Work out the finished part from the listing and answer in its coordinate system (mm). A direction names the side the tool comes from. Coordinates: 2 decimals unless noted, no trailing zeros. Write each loop counter-clockwise with the first axis right and the second up, starting at its lowest first coordinate (ties: lowest second). Pieces come first, ordered by that corner, then holes. Notation, with made-up numbers: (31, 35) - (72, 35) arc R11 ccw to (72, 48) - close; hole circle Ø3 at (58.5, 81). An arc over 180 degrees is marked (long way). One line per item, written item: value.
```python
from build123d import *

# Parameters (mm, degrees)
SKETCH2_W           = 40.6
SKETCH2_H           = 36.6
SKETCH2_W_2         = 6.4
SKETCH2_H_2         = 2.4
SKETCH2_W_3         = 5.8
SKETCH2_H_3         = 5.3
BOSS_EXTRUDE1_DEPTH = 19.8
CUT_EXTRUDE1_DEPTH  = 5.3
CUT_EXTRUDE2_DEPTH  = 30.3


with BuildPart() as part:
    # Sketch2 → Boss-Extrude1 (new body)
    with BuildSketch(Plane(origin=(0, 0, 0), x_dir=(0, 0, -1), z_dir=(1, 0, 0))):
        Rectangle(SKETCH2_W, SKETCH2_H)
        with Locations((-23.5, 9.8)):
            Rectangle(SKETCH2_W_2, SKETCH2_H_2)
        with Locations((9.9, 20.95)):
            Rectangle(SKETCH2_W_3, SKETCH2_H_3)
        with Locations((23.5, 9.8)):
            Rectangle(SKETCH2_W_2, SKETCH2_H_2)
    extrude(amount=BOSS_EXTRUDE1_DEPTH)

    # Sketch3 → Cut-Extrude1 (cut)
    with BuildSketch(Plane(origin=(0, 18.3, 0), x_dir=(1, 0, 0), z_dir=(0, 1, 0))):
        with BuildLine():
            Line((9.9, 7), (12.8, 7))
            Line((12.8, 7), (12.8, 9.9))
            ThreePointArc((12.8, 9.9), (11.950609665, 7.849390335), (9.9, 7))
        make_face()
        with BuildLine():
            ThreePointArc((9.9, 12.8), (11.950609665, 11.950609665), (12.8, 9.9))
            Line((12.8, 9.9), (12.8, 12.8))
            Line((12.8, 12.8), (9.9, 12.8))
        make_face()
        with BuildLine():
            ThreePointArc((7, 9.9), (7.849390335, 11.950609665), (9.9, 12.8))
            Line((9.9, 12.8), (7, 12.8))
            Line((7, 12.8), (7, 9.9))
        make_face()
        with BuildLine():
            Line((7, 7), (9.9, 7))
            ThreePointArc((9.9, 7), (7.849390335, 7.849390335), (7, 9.9))
            Line((7, 9.9), (7, 7))
        make_face()
        Polygon((0, 7), (7, 7), (7, 9.9), (7, 12.8), (0, 12.8), align=None)
        Polygon((12.8, 7), (19.8, 7), (19.8, 12.8), (12.8, 12.8), (12.8, 9.9), align=None)
    extrude(amount=CUT_EXTRUDE1_DEPTH, mode=Mode.SUBTRACT)

    # Sketch4 → Cut-Extrude2 (cut, through all)
    with BuildSketch(Plane(origin=(0, 11, 0), x_dir=(1, 0, 0), z_dir=(0, 1, 0))):
        with BuildLine():
            ThreePointArc((16.4, 25.877050983), (14.9, 26.45), (13.4, 25.877050983))
            Line((13.4, 25.877050983), (16.4, 25.877050983))
        make_face()
        with BuildLine():
            Line((16.4, 25.877050983), (13.4, 25.877050983))
            ThreePointArc((13.4, 25.877050983), (13.981441346, 22.146040409), (17.15, 24.2))
            ThreePointArc((17.15, 24.2), (16.953959591, 25.118558654), (16.4, 25.877050983))
        make_face()
        with BuildLine():
            Line((16.4, 26.7), (13.4, 26.7))
            Line((13.4, 26.7), (13.4, 25.877050983))
            ThreePointArc((13.4, 25.877050983), (14.9, 26.45), (16.4, 25.877050983))
            Line((16.4, 25.877050983), (16.4, 26.7))
        make_face()
        with BuildLine():
            ThreePointArc((7.15, 24.2), (6.953959591, 25.118558654), (6.4, 25.877050983))
            Line((6.4, 25.877050983), (3.4, 25.877050983))
            ThreePointArc((3.4, 25.877050983), (3.981441346, 22.146040409), (7.15, 24.2))
        make_face()
        with BuildLine():
            Line((3.4, 25.877050983), (6.4, 25.877050983))
            ThreePointArc((6.4, 25.877050983), (4.9, 26.45), (3.4, 25.877050983))
        make_face()
        with BuildLine():
            Line((6.4, 25.877050983), (6.4, 26.7))
            Line((6.4, 26.7), (3.4, 26.7))
            Line((3.4, 26.7), (3.4, 25.877050983))
            ThreePointArc((3.4, 25.877050983), (4.9, 26.45), (6.4, 25.877050983))
        make_face()
        with BuildLine():
            ThreePointArc((13.4, -25.877050983), (14.9, -26.45), (16.4, -25.877050983))
            Line((16.4, -25.877050983), (13.4, -25.877050983))
        make_face()
        with BuildLine():
            Line((13.4, -25.877050983), (16.4, -25.877050983))
            ThreePointArc((16.4, -25.877050983), (16.953959591, -25.118558654), (17.15, -24.2))
            ThreePointArc((17.15, -24.2), (13.981441346, -22.146040409), (13.4, -25.877050983))
        make_face()
        with BuildLine():
            Line((13.4, -26.7), (16.4, -26.7))
            Line((16.4, -26.7), (16.4, -25.877050983))
            ThreePointArc((16.4, -25.877050983), (14.9, -26.45), (13.4, -25.877050983))
            Line((13.4, -25.877050983), (13.4, -26.7))
        make_face()
        with BuildLine():
            ThreePointArc((3.4, -25.877050983), (4.9, -26.45), (6.4, -25.877050983))
            Line((6.4, -25.877050983), (3.4, -25.877050983))
        make_face()
        with BuildLine():
            Line((3.4, -25.877050983), (6.4, -25.877050983))
            ThreePointArc((6.4, -25.877050983), (6.953959591, -25.118558654), (7.15, -24.2))
            ThreePointArc((7.15, -24.2), (3.981441346, -22.146040409), (3.4, -25.877050983))
        make_face()
        with BuildLine():
            Line((3.4, -26.7), (6.4, -26.7))
            Line((6.4, -26.7), (6.4, -25.877050983))
            ThreePointArc((6.4, -25.877050983), (4.9, -26.45), (3.4, -25.877050983))
            Line((3.4, -25.877050983), (3.4, -26.7))
        make_face()
    extrude(amount=-CUT_EXTRUDE2_DEPTH, mode=Mode.SUBTRACT)


solid = part.part
```
Item 1: Section A-A, the plane x = 1.5 is taken. Determine the outline of the cut face in (y, z).
Evaluation:
outline: (-18.3, -20.3) - (8.6, -20.3) - (8.6, -26.7) - (11, -26.7) - (11, -20.3) - (18.3, -20.3) - (18.3, 20.3) - (11, 20.3) - (11, 26.7) - (8.6, 26.7) - (8.6, 20.3) - (-18.3, 20.3) - close
Item 2: Section C-C, the plane z = 12 is taken. Determine the outline of the cut face in (x, y), then the cut area to 3 significant figures.
Evaluation:
outline: (0, -18.3) - (19.8, -18.3) - (19.8, 18.3) - (0, 18.3) - close
area: 725 mm2
Item 3: Given pin 1 (4 mm diameter, centred on x = 7.5, y = 17, fed in from -Z); pin 2 (1.9 mm diameter, centred on x = 13, z = -23, fed in from +Y); pin 3 (10 mm diameter, centred on x = 9, z = 9.5, fed in from +Y), each flat-ended and moving along its own axis, determine where each tip first touches the part or whether it passes through.
Evaluation:
pin 1: stops at z = -20.3
pin 2: stops at y = 11
pin 3: stops at y = 18.3
Item 4: Section B-B, the plane y = 21 is taken. Determine the outline of the cut face in (x, z), then the cut area to 3 significant figures.
Evaluation:
outline: circle Ø5.8 at (9.9, -9.9)
area: 26.4 mm2
Item 5: Section D-D, the plane x = 14.9 is taken. Determine the outline of the cut face in (y, z).
Evaluation:
outline: (-18.3, -20.3) - (8.6, -20.3) - (8.6, -21.95) - (11, -21.95) - (11, -20.3) - (18.3, -20.3) - (18.3, 20.3) - (11, 20.3) - (11, 21.95) - (8.6, 21.95) - (8.6, 20.3) - (-18.3, 20.3) - close
Item 6: Consider probe 1 along X at (y, z) = (9.7, 24.2); probe 2 along Z at (x, y) = (10.5, -2.5); probe 3 along Z at (x, y) = (4.9, 9.75). Determine where each line is inside the solid, lowest interval first.
Evaluation:
probe 1: x = 0 to 2.65, 7.15 to 12.65, 17.15 to 19.8
probe 2: z = -20.3 to 20.3
probe 3: z = -21.95 to 21.95
Item 7: Which of the six approach directions +Z, -Z, +X, -X, +Y, -Y give full straight-line access (tool end or side, diameter ignored) to faces 1 (the face through (10, 8.6, 24)), 2 (the face through (10, 15, -20.3)), 3 (the face through (2, 10, -26.7)), 4 (the face through (10, 15, 20.3)), 5 (the face through (10, -5, -20.3))?
Evaluation:
face 1: +Z, +X, -X, -Y
face 2: -Z, +X, -X, +Y
face 3: -Z, +X, -X, +Y, -Y
face 4: +Z, +X, -X, +Y
face 5: -Z, +X, -X, -Y
